Could you check a few things on this drawing? It's one solid part, dimensions in mm from its lowest x, y, z. Coordinates: 2 decimals unless noted, no trailing zeros. Order: outer loops, then holes, each group sorted by start corner. A loop starts at its lowest first (then second) coordinate and runs counter-clockwise, first axis right, second up.
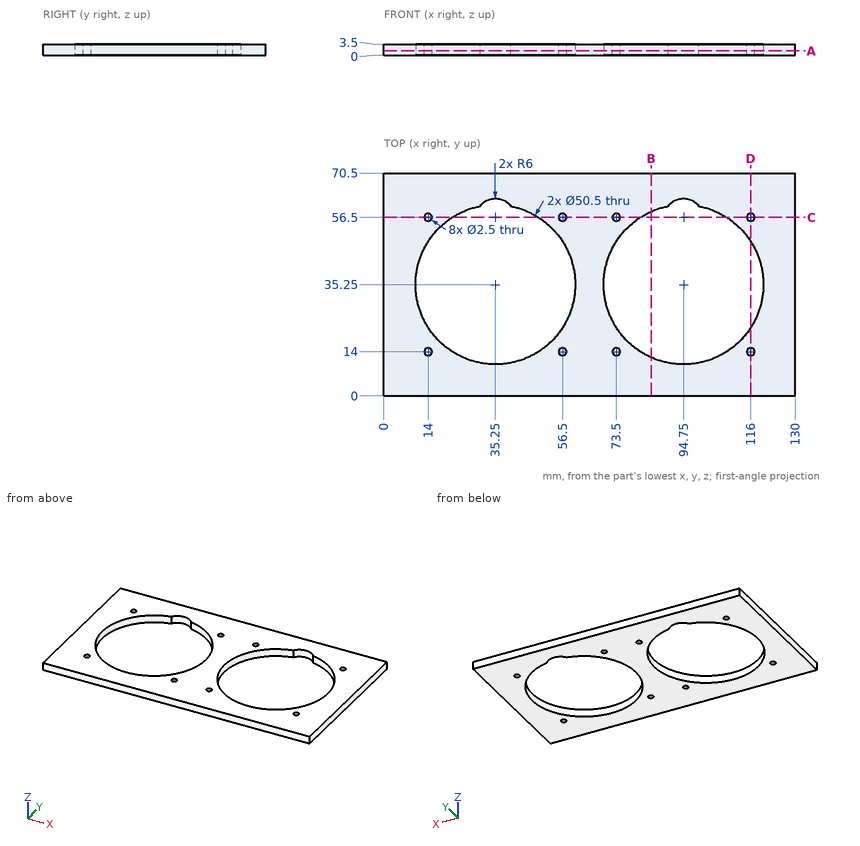
Q1. If we section it at A-A on z = 1.3: Give the number of separate pieces and of enclosed holes in the cut face, then the cut area to 3 significant figures.
Q2. Will this pin go through, and if not, where does the flat tip stop? pin 1 (4 mm diameter, centred on x = 116, y = 56.5, fed in from -Z).
Q3. I need wall thicknesses on L1, parallel to X at y = 29, z = 2.2; L2, parallel to X at y = 53.5, z = 0.65; L3, parallel to Y at x = 14.5, z = 2.8. Which ranges of each line are inside material? Lowest first, please.
Q4. If we section it at C-C on y = 56.5: Write out the boundary of the cut face in (x, z), then the cut area to 3 significant figures.
Q5. If we section it at B-B on x = 84.5: Write out the boundary of the cut face in (y, z), then the cut area to 3 significant figures.
Q6. If we section it at D-D on x = 116: Write out the boundary of the cut face in (y, z).
Reply:
1. separate pieces: 1
1. enclosed holes: 10
1. area: 5,090 mm2
2. pin 1: stops at z = 0
3. L1: x = 0 to 10.79, 59.71 to 70.29, 119.21 to 130
3. L2: x = 0 to 17.8, 52.7 to 77.3, 112.2 to 130
3. L3: y = 0 to 12.85, 15.15 to 20.86, 49.64 to 55.35, 57.65 to 70.5
4. outline: (0, 0) - (12.75, 0) - (12.75, 3.5) - (0, 3.5) - close; (15.25, 0) - (21.61, 0) - (21.61, 3.5) - (15.25, 3.5) - close; (48.89, 0) - (55.25, 0) - (55.25, 3.5) - (48.89, 3.5) - close; (57.75, 0) - (72.25, 0) - (72.25, 3.5) - (57.75, 3.5) - close; (74.75, 0) - (81.11, 0) - (81.11, 3.5) - (74.75, 3.5) - close; (108.39, 0) - (114.75, 0) - (114.75, 3.5) - (108.39, 3.5) - close; (117.25, 0) - (130, 0) - (130, 3.5) - (117.25, 3.5) - close
4. area: 229 mm2
5. outline: (0, 0) - (12.17, 0) - (12.17, 3.5) - (0, 3.5) - close; (58.33, 0) - (70.5, 0) - (70.5, 3.5) - (58.33, 3.5) - close
5. area: 85.2 mm2
6. outline: (0, 0) - (12.75, 0) - (12.75, 3.5) - (0, 3.5) - close; (15.25, 0) - (21.61, 0) - (21.61, 3.5) - (15.25, 3.5) - close; (48.89, 0) - (55.25, 0) - (55.25, 3.5) - (48.89, 3.5) - close; (57.75, 0) - (70.5, 0) - (70.5, 3.5) - (57.75, 3.5) - close
